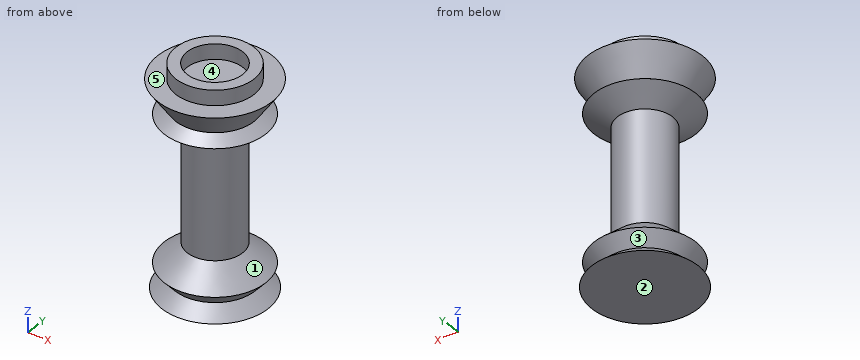
```python
from build123d import *

# Parameters (mm, degrees)
F0_W = 23.53953
F0_H = 31.575338


with BuildPart() as f1:
    # F0 (on Front) → F1 (revolve)
    with BuildSketch(Plane.XZ):
        Polygon((0, -342.900006), (0, 82.724656), (-58.029232, 82.724656), (-81.568762, 82.724656), (-119.018393, 82.724656), (-81.475385, 27.549231), (-105.595883, 11.136923), (-57.541642, -18.170769), (-57.541642, -250.007569), (-105.595883, -292.055042), (-82.647693, -318.281537), (-110.783078, -342.900006), align=None)
        with Locations((-69.798997, 98.512325)):
            Rectangle(F0_W, F0_H)
    revolve(axis=Axis((0, 0, -1.758462), (0, 0, -1)))


solid = f1.part
```
The listing builds one solid part. Answer for the finished solid, in the listing's coordinates (mm). Face numbers are marked on the shaded views. A direction names the side the tool comes from. Give positions to 0.01 mm unless a question says otherwise; leave off trailing zeros. Order: outer loops, then holes, each group sorted by start corner. A loop starts at its lowest first (then second) coordinate and runs counter-clockwise, first axis right, second up. Notation, with made-up numbers: (-28.75, -29.75) -> (-4.75, -29.75) arc R19 cw to (-4.75, 7.25) -> close; hole circle Ø5 at (62, -10.75). An arc over 180 degrees is marked (long way). Write each question's results on one line, items separated by ' | '.
Q1. Which of the six approach directions +Z, -Z, +X, -X, +Y, -Y give full straight-line access (tool end or side, diameter ignored) to the marked faces 1 and 2?
Checked values:
face 1: none | face 2: -Z, +X, -X, +Y, -Y
Q2. The part is cut by section A-A, the plane y = -97. State how many separate pieces and enclosed holes the cut face has, and give its area (3 significant figures).
Checked values:
separate pieces: 4 | enclosed holes: 0 | area: 5,330 mm^2
Q3. The part is cut by section C-C, the plane z = -32. Give the vertices of the cut face in (x, y).
Checked values:
outline: circle Ø115.08 at (0, 0)
Q4. The part is cut by section B-B, the plane x = 0. Give the vertices of the cut face in (y, z), and give its area (3 significant figures).
Checked values:
outline: (-119.02, 82.72) -> (-81.48, 27.55) -> (-105.6, 11.14) -> (-57.54, -18.17) -> (-57.54, -250.01) -> (-105.6, -292.06) -> (-82.65, -318.28) -> (-110.78, -342.9) -> (110.78, -342.9) -> (82.65, -318.28) -> (105.6, -292.06) -> (57.54, -250.01) -> (57.54, -18.17) -> (105.6, 11.14) -> (81.48, 27.55) -> (119.02, 82.72) -> (81.57, 82.72) -> (81.57, 114.3) -> (58.03, 114.3) -> (58.03, 82.72) -> (-58.03, 82.72) -> (-58.03, 114.3) -> (-81.57, 114.3) -> (-81.57, 82.72) -> close | area: 63,600 mm^2
Q5. Straight lines are drawn through the part: probe 1 along Y at (x, z) = (0, 97); probe 2 along Z at (x, y) = (-69.5, 78.5); probe 3 along Z at (x, y) = (92.5, 27). For each, find the intervals that lie inside material, in ascending order. Write a range as from..to.
Checked values:
probe 1: y = -81.57..-58.03, 58.03..81.57 | probe 2: z = -342.9..-337.7, -292.91..-291.4, 10.68..11.65, 61.89..82.72 | probe 3: z = -342.9..-330.28, -302.61..-283.97, 5.5..17.42, 49.42..82.72
Q6. Each of these flat-tipped pins is pushed along its axis until it touches: P1, Ø12, axis at x = 41.5, z = -169, coming from the +Y side; P2, Ø2, axis at x = 43.5, z = -166, coming from the -Y side; P3, Ø12, axis at y = 45.5, z = -206, coming from the -X side; P4, Ø8, axis at y = -64, z = -198, coming from the -X side. Where does it stop, or does it pass through?
Checked values:
P1: stops at y = 45.29 | P2: stops at y = -38.79 | P3: stops at x = -41.84 | P4: passes through
Q7. Determine the mould class of the marked faces 3, 4 and 5 for opening direction Y: pulls with the +Y half, pulls with the -Y half, needs draft (parallel to the pull), parting line crosses it, or undercut.
Checked values:
face 3: parting line crosses it | face 4: undercut | face 5: needs draft
